Design review of the part built by this model. Coordinates are the model's own, in mm. A direction names the side the tool comes from. Coordinates: 2 decimals unless noted, no trailing zeros. Write each loop counter-clockwise with the first axis right and the second up, starting at its lowest first coordinate (ties: lowest second). Pieces come first, ordered by that corner, then holes.
Q1. Machinability: for faces 1 (the cylindrical face through (-28.12, 2.54, -149.04)), 2 (the flat face through (-60, 4, -155)), which of the approach directions +Z, -Z, +X, -X, +Y, -Y give a long, thin tool a straight path to every point of the face, cutting with its end or side? Answer none if there is none.
Q2. Take a section at B-B (z = 16). Give the boundary of the cut face in (x, y).
Q3. Take a section at A-A (x = -90). Give the boundary of the cut face in (y, z), and give its area (3 significant figures).
Q4. For probe 1 along X at (y, z) = (2.6, 149.5); probe 2 along X at (y, z) = (3.3, -125); probe 3 along X at (y, z) = (2.15, -155), list the stretches that pass through material, from the lowest coordinate up.
Q5. Insertion check: pin 1 (5 mm diameter, centred on x = 147, z = -149.5, fed in from +Y); pin 2 (0.8 mm diameter, centred on y = 4.5, z = -148.5, fed in from +X); pin 3 (1 mm diameter, centred on y = 2, z = 149, fed in from -X); pin 4 (2.5 mm diameter, centred on x = 187, y = 2.5, fed in from +Z). Each pin has a flat end and moves straight along its axis. Give the tip position at first contact, or say it passes through.
Q6. Take a section at C-C (x = 60). Give the boundary of the cut face in (y, z), and give its area (3 significant figures).
Q7. Mouldability with a two-part tool opening along Z and no side actions: class faces 3 (the cylindrical face through (10.99, 2.46, -249.76)), 4 (the flat face through (4, 5, -3)), 5 (the flat face through (60, 4, -155)) as pulls with the +Z half, pulls with the -Z half, needs draft (parallel to the pull), parting line crosses it, or undercut.
Q8. Take a section at D-D (y = 1.4). State how many separate pieces and enclosed holes the cut face has, and give its area (3 significant figures).
```python
from build123d import *

# Parameters (mm, degrees)
SKETCH1_R                                 = 250
BOSS_EXTRUDE1_CICLE_BODY_DEPTH            = 5
SKETCH3_W                                 = 40
SKETCH3_H                                 = 140
CUT_DRIVE_WHEEL_DEPTH                     = 50
SKETCH5_R                                 = 1.5
SKETCH5_R_2                               = 5
CUT_DRIVE_WHEEL_FIXATION_DEPTH            = 10
SKETCH6_R                                 = 2
CUT_EXTRUDE_CASTER_WHEEEL_CUT_DEPTH       = 10
SKETCH7_R                                 = 6.25
SKETCH7_W                                 = 30
SKETCH7_H                                 = 30
CUT_EXTRUDE_EXTRUSION_FIXATION_BASE_DEPTH = 1
SKETCH9_R                                 = 6.25
CUT_EXTRUDE_1_25_BRACKET_HOLES_DEPTH      = 71


with BuildPart() as part:
    # Sketch1 → Boss-Extrude1_cicle body (new body)
    with BuildSketch(Plane(origin=(0, 0, 0), x_dir=(1, 0, 0), z_dir=(0, 1, 0))):
        with Locations(Location((0, 0, 0), (0, 0, 270))):
            Circle(SKETCH1_R)
    extrude(amount=BOSS_EXTRUDE1_CICLE_BODY_DEPTH)

    # Sketch3 → Cut-drive wheel (cut, symmetric)
    with BuildSketch(Plane(origin=(0, 0, 0), x_dir=(1, 0, 0), z_dir=(0, 1, 0))):
        with Locations((-190, 0)):
            Rectangle(SKETCH3_W, SKETCH3_H)
        with Locations((190, 0)):
            Rectangle(SKETCH3_W, SKETCH3_H)
    extrude(amount=CUT_DRIVE_WHEEL_DEPTH, both=True, mode=Mode.SUBTRACT)

    # Sketch5 → Cut- drive wheel_fixation (cut)
    with BuildSketch(Plane(origin=(0, 5, 0), x_dir=(1, 0, 0), z_dir=(0, 1, 0))):
        with Locations(Location((-162.40625, -8, 0), (0, 0, 270))):
            Circle(SKETCH5_R)
        with Locations(Location((-148.40625, 8, 0), (0, 0, 270))):
            Circle(SKETCH5_R)
        with Locations(Location((-155.40625, 0, 0), (0, 0, 270))):
            Circle(SKETCH5_R_2)
        with Locations(Location((-148.40625, -8, 0), (0, 0, 270))):
            Circle(SKETCH5_R)
        with Locations(Location((-162.40625, 8, 0), (0, 0, 270))):
            Circle(SKETCH5_R)
    cut_drive_wheel_fixation = extrude(amount=-CUT_DRIVE_WHEEL_FIXATION_DEPTH, mode=Mode.SUBTRACT)

    # Mirror-drive wheel: Cut- drive wheel_fixation across plane
    add(cut_drive_wheel_fixation.mirror(Plane(origin=(0, 0, 0), x_dir=(0, 0, 1), z_dir=(1, 0, 0))), mode=Mode.SUBTRACT)

    # Sketch6 → Cut-Extrude_caster_wheeel_cut (cut)
    with BuildSketch(Plane(origin=(0, 5, 0), x_dir=(1, 0, 0), z_dir=(0, 1, 0))):
        with Locations(Location((-123, 149.5, 0), (0, 0, 270))):
            Circle(SKETCH6_R)
        with Locations(Location((-147, 149.5, 0), (0, 0, 270))):
            Circle(SKETCH6_R)
        with Locations(Location((-147, 120.5, 0), (0, 0, 270))):
            Circle(SKETCH6_R)
        with Locations(Location((-123, 120.5, 0), (0, 0, 270))):
            Circle(SKETCH6_R)
        with Locations(Location((123, 149.5, 0), (0, 0, 270))):
            Circle(SKETCH6_R)
        with Locations(Location((147, 149.5, 0), (0, 0, 270))):
            Circle(SKETCH6_R)
        with Locations(Location((147, 120.5, 0), (0, 0, 270))):
            Circle(SKETCH6_R)
        with Locations(Location((123, 120.5, 0), (0, 0, 270))):
            Circle(SKETCH6_R)
        with Locations(Location((123, -149.5, 0), (0, 0, 270))):
            Circle(SKETCH6_R)
        with Locations(Location((123, -120.5, 0), (0, 0, 270))):
            Circle(SKETCH6_R)
        with Locations(Location((147, -149.5, 0), (0, 0, 270))):
            Circle(SKETCH6_R)
        with Locations(Location((147, -120.5, 0), (0, 0, 270))):
            Circle(SKETCH6_R)
        with Locations(Location((-123, -120.5, 0), (0, 0, 270))):
            Circle(SKETCH6_R)
        with Locations(Location((-147, -120.5, 0), (0, 0, 270))):
            Circle(SKETCH6_R)
        with Locations(Location((-147, -149.5, 0), (0, 0, 270))):
            Circle(SKETCH6_R)
        with Locations(Location((-123, -149.5, 0), (0, 0, 270))):
            Circle(SKETCH6_R)
    extrude(amount=-CUT_EXTRUDE_CASTER_WHEEEL_CUT_DEPTH, mode=Mode.SUBTRACT)

    # Sketch7 → Cut-Extrude__extrusion_fixation_base (cut)
    with BuildSketch(Plane(origin=(0, 5, 0), x_dir=(1, 0, 0), z_dir=(0, 1, 0))):
        with Locations(Location((-90, 155, 0), (0, 0, 270))):
            Circle(SKETCH7_R)
        with Locations(Location((-60, 185, 0), (0, 0, 270))):
            Circle(SKETCH7_R)
        with Locations(Location((-30, 155, 0), (0, 0, 270))):
            Circle(SKETCH7_R)
        with Locations(Location((-60, 125, 0), (0, 0, 270))):
            Circle(SKETCH7_R)
        with Locations(Location((90, 155, 0), (0, 0, 90))):
            Circle(SKETCH7_R)
        with Locations(Location((60, 125, 0), (0, 0, 90))):
            Circle(SKETCH7_R)
        with Locations(Location((30, 155, 0), (0, 0, 90))):
            Circle(SKETCH7_R)
        with Locations(Location((60, 185, 0), (0, 0, 90))):
            Circle(SKETCH7_R)
        with Locations((60, 155)):
            Rectangle(SKETCH7_W, SKETCH7_H)
        with Locations((-60, 155)):
            Rectangle(SKETCH7_W, SKETCH7_H)
    extrude(amount=-CUT_EXTRUDE_EXTRUSION_FIXATION_BASE_DEPTH, mode=Mode.SUBTRACT)

    # Sketch9 → Cut-Extrude_1.25 bracket holes (cut)
    with BuildSketch(Plane(origin=(0, 4, 0), x_dir=(1, 0, 0), z_dir=(0, 1, 0))):
        with Locations(Location((-60, 185, 0), (0, 0, 270))):
            Circle(SKETCH9_R)
        with Locations(Location((-30, 155, 0), (0, 0, 270))):
            Circle(SKETCH9_R)
        with Locations(Location((-90, 155, 0), (0, 0, 270))):
            Circle(SKETCH9_R)
        with Locations(Location((-60, 125, 0), (0, 0, 270))):
            Circle(SKETCH9_R)
        with Locations(Location((60, 185, 0), (0, 0, 270))):
            Circle(SKETCH9_R)
        with Locations(Location((30, 155, 0), (0, 0, 270))):
            Circle(SKETCH9_R)
        with Locations(Location((60, 125, 0), (0, 0, 270))):
            Circle(SKETCH9_R)
        with Locations(Location((90, 155, 0), (0, 0, 270))):
            Circle(SKETCH9_R)
    extrude(amount=-CUT_EXTRUDE_1_25_BRACKET_HOLES_DEPTH, mode=Mode.SUBTRACT)


solid = part.part
```
Response:
1. face 1: +Y, -Y
1. face 2: +Y
2. outline: (-249.49, 0) - (-210, 0) - (-210, 5) - (-249.49, 5) - close; (-170, 0) - (170, 0) - (170, 5) - (-170, 5) - close; (210, 0) - (249.49, 0) - (249.49, 5) - (210, 5) - close
3. outline: (0, -233.24) - (5, -233.24) - (5, -161.25) - (0, -161.25) - close; (0, -148.75) - (5, -148.75) - (5, 233.24) - (0, 233.24) - close
3. area: 2,270 mm2
4. probe 1: x = -200.37 to -149, -145 to -125, -121 to 121, 125 to 145, 149 to 200.37
4. probe 2: x = -216.51 to -66.25, -53.75 to 53.75, 66.25 to 216.51
4. probe 3: x = -196.15 to -96.25, -83.75 to -36.25, -23.75 to 23.75, 36.25 to 83.75, 96.25 to 196.15
5. pin 1: stops at y = 5
5. pin 2: stops at x = 201.41
5. pin 3: stops at x = -201.12
5. pin 4: stops at z = 167.32
6. outline: (0, -242.69) - (5, -242.69) - (5, -191.25) - (0, -191.25) - close; (0, -178.75) - (5, -178.75) - (5, -170) - (4, -170) - (4, -140) - (5, -140) - (5, -131.25) - (0, -131.25) - close; (0, -118.75) - (5, -118.75) - (5, 242.69) - (0, 242.69) - close
6. area: 2,270 mm2
7. face 3: parting line crosses it
7. face 4: needs draft
7. face 5: undercut
8. separate pieces: 1
8. enclosed holes: 36
8. area: 184,000 mm2
